Work out the finished part from the listing and answer in its coordinate system (mm). Face numbers are marked on the shaded views. A direction names the side the tool comes from. Round coordinates to 2 decimals unless told otherwise and drop trailing zeros. Loops run counter-clockwise (first coordinate to the right, second up) from the corner with the lowest first, then second, coordinate; pieces in that order, holes last.
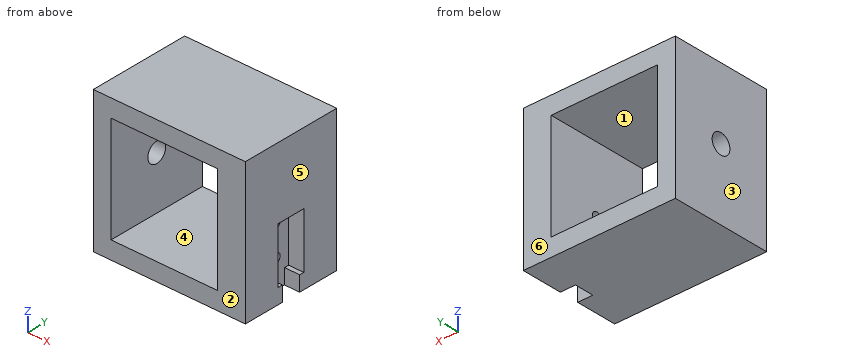
Autodesk Inventor part; units mm, degrees
ref_plane "YZ Plane" through (0, 0, 0) normal (1, 0, 0) x (0, 1, 0)
ref_plane "XZ Plane" through (0, 0, 0) normal (0, 1, 0) x (-1, 0, 0)
ref_plane "XY Plane" through (0, 0, 0) normal (0, 0, 1) x (1, 0, 0)
sketch "Sketch1" plane through (0, 0, 0) normal (0, 1, 0) x (-1, 0, 0)
  line L0 (-10.5, -10.5) -> (10.5, -10.5)
  line L1 (10.5, -10.5) -> (10.5, 10.5)
  line L2 (10.5, 10.5) -> (-10.5, 10.5)
  line L3 (-10.5, 10.5) -> (-10.5, -10.5)
  line L4 (-10.5, -10.5) -> (10.5, 10.5) construction
  line L5 (10.5, -10.5) -> (-10.5, 10.5) construction
  line L6 (-14, -14) -> (14, -14)
  line L7 (14, -14) -> (14, 14)
  line L8 (14, 14) -> (-14, 14)
  line L9 (-14, -14) -> (14, 14) construction
  line L10 (14, -14) -> (-14, 14) construction
  line L11 (-14, 14) -> (-16, 14)
  line L12 (-14, -14) -> (-16, -14)
  line L13 (-16, -14) -> (-16, 14)
  line L14 (-14, 14) -> (-14, 10.5)
  line L15 (-14, -10.5) -> (-14, -14)
  point P0 (0, 0)
  dimension "d0" = 21
  dimension "d1" = 21
  dimension "d2" = 28
  dimension "d3" = 28
  dimension "d6" = 2
extrude "Extrusion1" add sketch "Sketch1" along normal blind 20
sketch "Sketch3" plane through (16, 0, 14) normal (1, 0, 0) x (0, 0, -1)
  line L0 (28, 0) -> (28, 20)
  line L1 (28, 10) -> (0, 10) construction
  line L2 (0, 0) -> (0, 20)
  line L3 (14, 10) -> (14, 12.8)
  line L4 (14, 12.8) -> (25, 12.8)
  line L5 (14, 10) -> (14, 7.2)
  line L6 (14, 7.2) -> (25, 7.2)
  line L7 (28, 11.9) -> (25, 11.9)
  line L8 (25, 8.1) -> (28, 8.1)
  line L9 (25, 11.9) -> (25, 12.8)
  line L10 (25, 8.1) -> (25, 7.2)
  point P0 (14, 0)
  dimension "d7" = 2.8
  dimension "d8" = 2.8
  dimension "d10" = 3
  dimension "d24" = 1.9
  dimension "d25" = 1.9
extrude "Extrusion2" cut sketch "Sketch3" against normal blind 3
sketch "Sketch4" plane through (13, 0, 14) normal (1, 0, 0) x (0, 0, -1)
  line L0 (28, 11.9) -> (28, 8.1)
  line L1 (28, 10) -> (14, 10) construction
  circle A0 centre (22.5, 10) radius 0.95
  circle A1 centre (16.5, 10) radius 0.95
  line L2 (14, 7.2) -> (14, 12.8)
  point P0 (14, 0)
  dimension "d14" = 1.9
  dimension "d15" = 1.9
  dimension "d16" = 6
  dimension "d22" = 2.5
extrude "Extrusion3" cut sketch "Sketch4" against normal blind 3
sketch "Sketch5" plane through (-14, 0, -14) normal (-1, 0, 0) x (0, 0, 1)
  line L0 (14, 7.2) -> (14, 12.8)
  circle A0 centre (14, 10) radius 1.95
  point P0 (14, 0)
  dimension "d19" = 3.9
extrude "Extrusion4" cut sketch "Sketch5" against normal blind 4
properties part number "holder"
1. Consider probe 1 along Z at (x, y) = (-3, 2); probe 2 along Y at (x, z) = (11.45, -8.5); probe 3 along X at (y, z) = (15.75, -3.5). Determine where each line is inside the solid, lowest interval first.
Answer key:
probe 1: z = -14 to -10.5, 10.5 to 14
probe 2: y = 0 to 9.05, 10.95 to 20
probe 3: x = -14 to -10.5, 10.5 to 16
2. Find section D-D (y = 15.25). Write down the section's boundary in (x, z).
Answer key:
outline: (-14, -14) - (16, -14) - (16, 14) - (-14, 14) - close; hole (-10.5, -10.5) - (10.5, -10.5) - (10.5, 10.5) - (-10.5, 10.5) - close
3. Find section A-A (x = 1). Write down the section's boundary in (y, z), then the cut area to 3 significant figures.
Answer key:
outline: (0, -14) - (20, -14) - (20, -10.5) - (0, -10.5) - close; (0, 10.5) - (20, 10.5) - (20, 14) - (0, 14) - close
area: 140 mm2
4. Find section C-C (z = -5). Write down the section's boundary in (x, y).
Answer key:
outline: (-14, 0) - (-10.5, 0) - (-10.5, 20) - (-14, 20) - close; (10.5, 0) - (16, 0) - (16, 7.2) - (13, 7.2) - (13, 12.8) - (16, 12.8) - (16, 20) - (10.5, 20) - close
5. Which of the six approach directions +Z, -Z, +X, -X, +Y, -Y give full straight-line access (tool end or side, diameter ignored) to the marked faces 1 and 2?
Answer key:
face 1: +Y, -Y
face 2: +Z, -Z, +X, -X, -Y
6. Find section B-B (y = 10). Write down the section's boundary in (x, z), then the cut area to 3 significant figures.
Answer key:
outline: (-14, -14) - (13, -14) - (13, -9.45) - (10.5, -9.45) - (10.5, -10.5) - (-10.5, -10.5) - (-10.5, -1.95) - (-14, -1.95) - close; (-14, 1.95) - (-10.5, 1.95) - (-10.5, 10.5) - (10.5, 10.5) - (10.5, -1.55) - (13, -1.55) - (13, 0) - (16, 0) - (16, 14) - (-14, 14) - close; (10.5, -7.55) - (13, -7.55) - (13, -3.45) - (10.5, -3.45) - close
area: 334 mm2
7. Determine the mould class of the marked faces 3, 4, 5 and 6 for opening direction X: +X half, -X half, draft (parallel to the pull), parting line (faces both ways), or undercut.
Answer key:
face 3: -X half
face 4: undercut
face 5: +X half
face 6: draft
8. Given pin 1 (1.7 mm diameter, centred on y = 11, z = -3.5, fed in from +X); pin 2 (0.9 mm diameter, centred on x = 14.5, y = 9.5, fed in from -Z); pin 3 (3.5 mm diameter, centred on y = 10, z = 0, fed in from -X); pin 4 (6 mm diameter, centred on x = -5, z = -7, fed in from +Y), each flat-ended and moving along its own axis, determine where each tip first touches the part or whether it passes through.
Answer key:
pin 1: stops at x = 13
pin 2: stops at z = 0
pin 3: stops at x = 10.5
pin 4: passes through
